Build history of the part. All positions in model axes, mm. Face numbers are marked on the shaded views. A direction names the side the tool comes from. Give positions to 0.01 mm unless a question says otherwise; leave off trailing zeros. Loops run counter-clockwise (first coordinate to the right, second up) from the corner with the lowest first, then second, coordinate; pieces in that order, holes last. Notation, with made-up numbers: (-5.5, 82) - (21.5, 82) arc R26 ccw to (21.5, 112) - close; hole circle Ø9 at (-5, 40.5). An arc over 180 degrees is marked (long way). Return JSON: item names as keys, results as strings. Group by question number.
1) Slice it at D-D (x = -263). List the corners of the cut face in (y, z) (3 decimals).
2) Slice it at B-B (y = 90). List the corners of the cut face in (x, z) (1 decimal).
3) 3-axis set-ups, long thin cutter, end or side, ignore diameter. For the marked faces 4 and 5: which of +Z, -Z, +X, -X, +Y, -Y reach the whole face in a straight line?
4) Drill centre lines: probe 1 along X at (y, z) = (9, 0) (3 decimals); probe 2 along Y at (x, z) = (-9, 0); probe 3 along Z at (x, y) = (-165.1, 12.5) (3 decimals). Where is each one in solid material? Low to high. Write a range as from..to.
5) Drop flat-ended pins along their axis: pin 1 (1.9 mm diameter, centred on y = 100, z = 1, fed in from +X); pin 2 (1 mm diameter, centred on x = -210.5, z = -7, fed in from +Y); pin 3 (3 mm diameter, centred on x = -166, z = -1, fed in from -Y). Give the stop position or say it passes through.
6) Slice it at A-A (y = 14). List the corners of the cut face in (x, z) (3 decimals), and give its area (3 significant figures).
7) Slice it at C-C (x = -66). List the corners of the cut face in (y, z) (3 decimals), and give its area (3 significant figures).
8) Mould opens along X. For the marked faces 1, 2 and 3 say: released by +X, released by -X, zero draft, split by the parting line, or undercut.
```python
from build123d import *

# Parameters (mm, degrees)
BOSS_EXTRUDE1_DEPTH              = 9.525
F_1_4_20_TAPPED_HOLE3_AT_2_COUNT = 2
F_1_4_20_TAPPED_HOLE3_AT_2_PITCH = 38.1
F_1_4_20_TAPPED_HOLE3_AT_3_COUNT = 2
F_1_4_20_TAPPED_HOLE3_AT_3_PITCH = 76.2
F_1_4_20_TAPPED_HOLE3_AT_4_COUNT = 2
F_1_4_20_TAPPED_HOLE3_AT_4_PITCH = 114.3
F_1_4_20_TAPPED_HOLE2_AT_2_COUNT = 2
F_1_4_20_TAPPED_HOLE2_AT_2_PITCH = 76.2
F_1_4_20_TAPPED_HOLE2_AT_3_COUNT = 2
F_1_4_20_TAPPED_HOLE2_AT_3_PITCH = 152.4
F_1_4_20_TAPPED_HOLE2_AT_4_COUNT = 2
F_1_4_20_TAPPED_HOLE2_AT_4_PITCH = 228.6
F_1_4_20_TAPPED_HOLE2_AT_5_COUNT = 2
F_1_4_20_TAPPED_HOLE2_AT_5_PITCH = 304.8


with BuildPart() as part:
    # Sketch1 w/mock PCB → Boss-Extrude1 (new body, symmetric)
    with BuildSketch(Plane.XY):
        Polygon((-19.05, 148.59), (-330.2, 21.59), (-330.2, 2.54), (0, 2.54), (0, 148.59), align=None)
        with BuildLine():
            Line((-25.4, 99.663010652), (-25.4, 40.64))
            ThreePointArc((-25.4, 40.64), (-29.119743879, 31.659743879), (-38.1, 27.94))
            Line((-38.1, 27.94), (-182.706376097, 27.94))
            ThreePointArc((-182.706376097, 27.94), (-195.168718703, 38.194592718), (-187.505667965, 52.398265075))
            Line((-187.505667965, 52.398265075), (-42.899291867, 111.421275727))
            ThreePointArc((-42.899291867, 111.421275727), (-31.016957106, 110.20438169), (-25.4, 99.663010652))
        make_face(mode=Mode.SUBTRACT)
    extrude(amount=BOSS_EXTRUDE1_DEPTH, both=True)

    # Sketch6 → 1/4-20 Tapped Hole3 (revolve, cut)
    with BuildSketch(Plane(origin=(0, 139.065, 0), x_dir=(0, 0, -1), z_dir=(0, 1, 0))):
        Polygon((0, 0), (0, 20.583816902), (2.5527, 19.05), (2.5527, 17.78), (3.175, 17.78), (3.175, 0.127), (3.302, 0), align=None)
    f_1_4_20_tapped_hole3 = revolve(axis=Axis((6.35, 139.065, 0), (-1, 0, 0)), mode=Mode.SUBTRACT)

    # 1/4-20 Tapped Hole3 at 2: 1/4-20 Tapped Hole3 ×2
    with Locations(*[(0, -i * F_1_4_20_TAPPED_HOLE3_AT_2_PITCH, 0) for i in range(1, F_1_4_20_TAPPED_HOLE3_AT_2_COUNT)]):
        add(f_1_4_20_tapped_hole3, mode=Mode.SUBTRACT)

    # 1/4-20 Tapped Hole3 at 3: 1/4-20 Tapped Hole3 ×2
    with Locations(*[(0, -i * F_1_4_20_TAPPED_HOLE3_AT_3_PITCH, 0) for i in range(1, F_1_4_20_TAPPED_HOLE3_AT_3_COUNT)]):
        add(f_1_4_20_tapped_hole3, mode=Mode.SUBTRACT)

    # 1/4-20 Tapped Hole3 at 4: 1/4-20 Tapped Hole3 ×2
    with Locations(*[(0, -i * F_1_4_20_TAPPED_HOLE3_AT_4_PITCH, 0) for i in range(1, F_1_4_20_TAPPED_HOLE3_AT_4_COUNT)]):
        add(f_1_4_20_tapped_hole3, mode=Mode.SUBTRACT)

    # Sketch8 → 1/4-20 Tapped Hole2 (revolve, cut)
    with BuildSketch(Plane(origin=(-12.7, 2.54, 0), x_dir=(0, 0, -1), z_dir=(1, 0, 0))):
        Polygon((0, 0), (0, 20.583816902), (2.5527, 19.05), (2.5527, 17.78), (3.175, 17.78), (3.175, 0.127), (3.302, 0), align=None)
    f_1_4_20_tapped_hole2 = revolve(axis=Axis((-12.7, -3.81, 0), (0, 1, 0)), mode=Mode.SUBTRACT)

    # 1/4-20 Tapped Hole2 at 2: 1/4-20 Tapped Hole2 ×2
    with Locations(*[(-i * F_1_4_20_TAPPED_HOLE2_AT_2_PITCH, 0, 0) for i in range(1, F_1_4_20_TAPPED_HOLE2_AT_2_COUNT)]):
        add(f_1_4_20_tapped_hole2, mode=Mode.SUBTRACT)

    # 1/4-20 Tapped Hole2 at 3: 1/4-20 Tapped Hole2 ×2
    with Locations(*[(-i * F_1_4_20_TAPPED_HOLE2_AT_3_PITCH, 0, 0) for i in range(1, F_1_4_20_TAPPED_HOLE2_AT_3_COUNT)]):
        add(f_1_4_20_tapped_hole2, mode=Mode.SUBTRACT)

    # 1/4-20 Tapped Hole2 at 4: 1/4-20 Tapped Hole2 ×2
    with Locations(*[(-i * F_1_4_20_TAPPED_HOLE2_AT_4_PITCH, 0, 0) for i in range(1, F_1_4_20_TAPPED_HOLE2_AT_4_COUNT)]):
        add(f_1_4_20_tapped_hole2, mode=Mode.SUBTRACT)

    # 1/4-20 Tapped Hole2 at 5: 1/4-20 Tapped Hole2 ×2
    with Locations(*[(-i * F_1_4_20_TAPPED_HOLE2_AT_5_PITCH, 0, 0) for i in range(1, F_1_4_20_TAPPED_HOLE2_AT_5_COUNT)]):
        add(f_1_4_20_tapped_hole2, mode=Mode.SUBTRACT)


solid = part.part
```
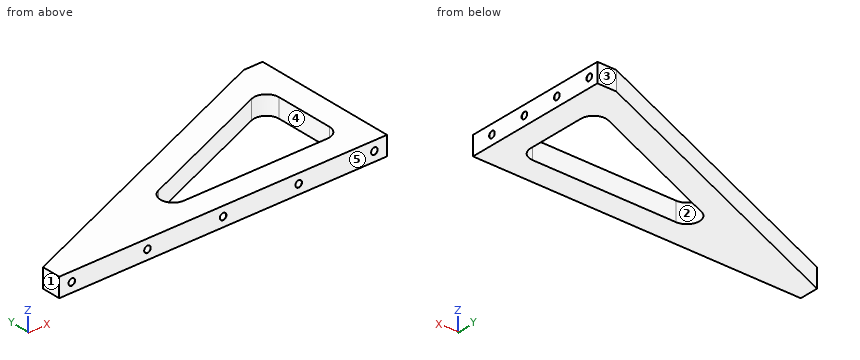
Results:
{
 "1": {"outline": "(2.54, -9.525) - (49.019, -9.525) - (49.019, 9.525) - (2.54, 9.525) - close"},
 "2": {"outline": "(-162.6, -9.5) - (-95.4, -9.5) - (-95.4, 9.5) - (-162.6, 9.5) - close; (-25.4, -9.5) - (0, -9.5) - (0, 9.5) - (-25.4, 9.5) - close"},
 "3": {"face 4": "+Z, -Z", "face 5": "+Z, -Z, +X, -X, -Y"},
 "4": {"probe 1": "-330.2..-320.675, -314.325..-244.475, -238.125..-168.275, -161.925..-92.075, -85.725..-15.875, -9.525..0", "probe 2": "2.54..21.59, 27.94..59.69, 66.04..97.79, 104.14..135.89, 142.24..148.59", "probe 3": "-9.525..-3.175, 3.175..9.525"},
 "5": {"pin 1": "x = -19.18", "pin 2": "y = 70.65", "pin 3": "y = 20.32"},
 "6": {"outline": "(-330.2, -9.525) - (0, -9.525) - (0, 9.525) - (-330.2, 9.525) - close; hole circle Ø6.35 at (-317.5, 0); hole circle Ø6.35 at (-241.3, 0); hole circle Ø6.35 at (-165.1, 0); hole circle Ø6.35 at (-88.9, 0); hole circle Ø6.35 at (-12.7, 0)", "area": "6,130 mm2"},
 "7": {"outline": "(2.54, -9.525) - (27.94, -9.525) - (27.94, 9.525) - (2.54, 9.525) - close; (101.992, -9.525) - (129.427, -9.525) - (129.427, 9.525) - (101.992, 9.525) - close", "area": "1,010 mm2"},
 "8": {"face 1": "released by -X", "face 2": "undercut", "face 3": "zero draft"}
}
